Geometry: final body of the model. Coordinates: model frame, mm. A direction names the side the tool comes from. Coordinates: 2 decimals unless noted, no trailing zeros. Order: outer loops, then holes, each group sorted by start corner. A loop starts at its lowest first (then second) coordinate and runs counter-clockwise, first axis right, second up. Notation, with made-up numbers: (-30, 56.25) -> (19, 56.25) arc R31 cw to (19, 91.25) -> close; hole circle Ø4 at (78, 50). An arc over 180 degrees is marked (long way). Answer in a Markdown table with one row per item. Add a question column.
1) Ray query, line 1 (Y direction, x = 119.5, z = -6.5); line 2 (X direction, y = 43, z = -23); line 3 (X direction, y = 11, z = -4). Return the intervals inside material, ascending. Write a range as from..to.
2) Section query A-A on y = 8. Return the cut outline in (x, z).
3) Contact query for a flat-ended pin moving along its axis: P1, Ø3, axis at x = 116.5, z = -7.5, coming from the -Y side. Output: stop coordinate, or through.
4) Set-up query: faces 4 (the face through (116, 29, 0)), 5 (the face through (112.57, 8.22, -12.4)), 6 (the face through (120.076, 8.217, -12.744)). Return all of +Z, -Z, +X, -X, +Y, -Y with unobstructed straight access to the full face (end or side cutting, diameter ignored); none if empty.
5) Section query C-C on z = -2.75. Return the cut outline in (x, y), then the cut area to 3 significant figures.
6) Section query B-B on z = -9.75. Return the cut outline in (x, y).
7) Pull-direction query (Z, two-part tool) for faces 1 (the face through (116, 29, -25)), 2 (the face through (115.1, 42.425, -19.965)), 3 (the face through (121, 0, -15)); classes: +Z half, -Z half, draft (parallel to the pull), parting line (faces both ways), or undercut.
```python
from build123d import *

# Parameters (mm, degrees)
SKETCH1_W           = 15
SKETCH1_H           = 25
BOSS_EXTRUDE1_DEPTH = 42
CUT_EXTRUDE1_DEPTH  = 16.666666667
SKETCH3_W           = 15
SKETCH3_H           = 25
BOSS_EXTRUDE2_DEPTH = 6.25
CUT_EXTRUDE2_REACH  = 136.927
SKETCH5_R           = 2.25


with BuildPart() as part:
    # Sketch1 → Boss-Extrude1 (new body)
    with BuildSketch(Plane(origin=(0, 0, 0), x_dir=(1, 0, 0), z_dir=(0, 1, 0))):
        with Locations((116, 12.5)):
            Rectangle(SKETCH1_W, SKETCH1_H)
    extrude(amount=BOSS_EXTRUDE1_DEPTH)

    # Sketch2 → Cut-Extrude1 (cut)
    with BuildSketch(Plane(origin=(0, 0, 0), x_dir=(1, 0, 0), z_dir=(0, 1, 0))):
        with BuildLine():
            Line((110.45615646, 25), (118.133663703, 25))
            ThreePointArc((118.133663703, 25), (120.094134728, 12.568265748), (120.75, 0))
            Line((120.75, 0), (113.25, 0))
            ThreePointArc((113.25, 0), (112.549371875, 12.57781342), (110.45615646, 25))
        make_face()
    extrude(amount=CUT_EXTRUDE1_DEPTH, mode=Mode.SUBTRACT)

    # Sketch3 → Boss-Extrude2 (add)
    with BuildSketch(Plane(origin=(0, 42, 0), x_dir=(1, 0, 0), z_dir=(0, 1, 0))):
        with Locations((116, 12.5)):
            Rectangle(SKETCH3_W, SKETCH3_H)
    extrude(amount=BOSS_EXTRUDE2_DEPTH)

    # Cut-Extrude2: up to this plane
    cut_extrude2_end = Plane(origin=(0, 48.25, 0), z_dir=(0, -1, 0))
    # Sketch5 → Cut-Extrude2 (cut, up to the surface)
    with BuildSketch(Plane(origin=(0, 0, 0), x_dir=(0.7071067811865464, 0, -0.7071067811865488), z_dir=(0.577381545199981, 0.5772877120855483, 0.577381545199979)), mode=Mode.PRIVATE) as cut_extrude2_sk1:
        with Locations(Location((95, -2, 0), (0, 0, 105.498899772))):
            Circle(SKETCH5_R)
    cut_extrude2_tool1 = split(extrude(cut_extrude2_sk1.sketch, amount=CUT_EXTRUDE2_REACH, mode=Mode.PRIVATE), bisect_by=cut_extrude2_end, keep=Keep.BOTH, mode=Mode.PRIVATE)
    add(cut_extrude2_tool1.solids().sort_by_distance((67.991552, -1.633082, -66.358736))[0], mode=Mode.SUBTRACT)


solid = part.part
```
Result:
| question | item | result |
|---|---|---|
| 1 | line 1 | 16.67..48.25 |
| 1 | line 2 | 108.5..109.47, 114.51..123.5 |
| 1 | line 3 | 108.5..113.18, 120.68..123.5 |
| 2 | outline | (108.5, -25) -> (110.46, -25) arc R113.25 ccw to (113.25, 0) -> (108.5, 0) -> close; (118.13, -25) -> (123.5, -25) -> (123.5, 0) -> (120.75, 0) arc R120.75 cw to start |
| 3 | P1 | y = 16.67 |
| 4 | face 4 | +Z, +X, -X, +Y, -Y |
| 4 | face 5 | -Z, -Y |
| 4 | face 6 | +Z, -Y |
| 5 | outline | (108.5, 0) -> (113.22, 0) -> (113.22, 16.67) -> (120.72, 16.67) -> (120.72, 0) -> (123.5, 0) -> (123.5, 48.25) -> (108.5, 48.25) -> close |
| 5 | area | 599 mm2 |
| 6 | outline | (108.5, 0) -> (112.83, 0) -> (112.83, 16.67) -> (120.36, 16.67) -> (120.36, 0) -> (123.5, 0) -> (123.5, 48.25) -> (108.5, 48.25) -> close |
| 7 | face 1 | -Z half |
| 7 | face 2 | undercut |
| 7 | face 3 | draft |
